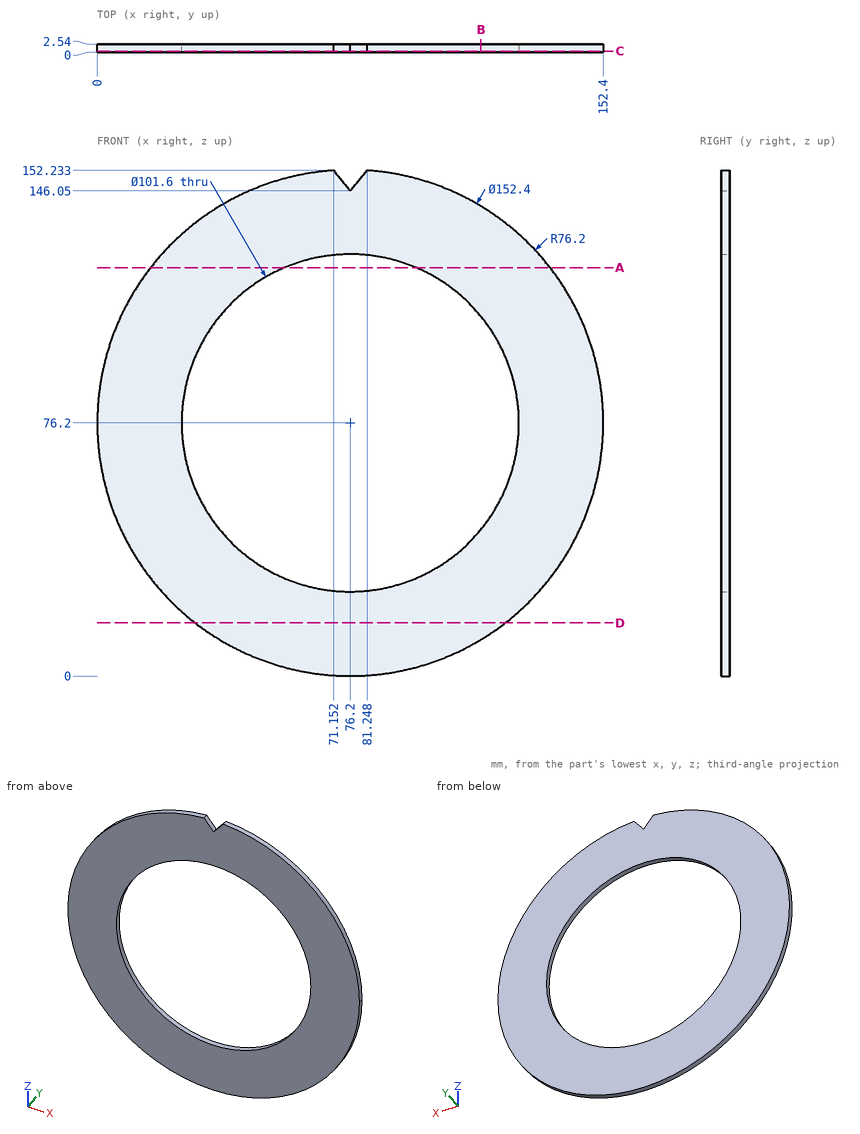
Print and shaded views of the part. All mm, measured from the part's lowest x, y and z. Round coordinates to 2 decimals unless told otherwise and drop trailing zeros. Write each loop counter-clockwise with the first axis right and the second up, starting at its lowest first coordinate (ties: lowest second). Pieces come first, ordered by that corner, then holes. Notation, with made-up numbers: (29.5, 82) - (84.5, 82) arc R32 cw to (84.5, 112) - close; hole circle Ø11 at (29, -17.5). An arc over 180 degrees is marked (long way). Use CSV: the item, a comma, the result in double quotes. Start each with the question number.
Item 1: Band-saw the part on A-A (z = 123). Write the cut outline in (x, y) (1 decimal).
Item 2: Band-saw the part on C-C (y = 0.4). Write the cut outline in (x, z), and give its area (3 significant figures).
Item 3: Band-saw the part on B-B (x = 115.5). Write the cut outline in (y, z).
Item 4: Drill centre lines: L1, parallel to Z at x = 76.2, y = 1.45; L2, parallel to X at y = 1.2, z = 118; L3, parallel to X at y = 1.55, z = 33.5 (1 decimal). Where is each one in solid material? Low to high. Write a range as [from, to].
Item 5: Band-saw the part on D-D (z = 16). Write the cut outline in (x, y), and give its area (3 significant figures).
Item 6: Pin check, flat tips, straight feed: P1, Ø1.5, axis at y = 0.5, z = 54.5, coming from the -X side; P2, Ø1.5, axis at x = 126.5, y = 1, coming from the +Z side; P3, Ø10, axis at x = 93.5, z = 115, coming from the +Y side. Stop position of each tip, or through.
Checked values:
1,outline,"(16.1, 0) - (56.4, 0) - (56.4, 2.5) - (16.1, 2.5) - close; (96, 0) - (136.3, 0) - (136.3, 2.5) - (96, 2.5) - close"
2,outline,"(71.15, 152.23) arc R76.2 ccw (long way) to (81.25, 152.23) - (76.2, 146.05) - close; hole circle Ø101.6 at (76.2, 76.2)"
2,area,"10,100 mm²"
3,outline,"(0, 10.92) - (2.54, 10.92) - (2.54, 44.01) - (0, 44.01) - close; (0, 108.39) - (2.54, 108.39) - (2.54, 141.48) - (0, 141.48) - close"
4,L1,"z = [0, 25.4], [127, 146.05]"
4,L2,"x = [12.49, 47.33], [105.07, 139.91]"
4,L3,"x = [13.1, 48.7], [103.7, 139.3]"
5,outline,"(29.48, 0) - (122.92, 0) - (122.92, 2.54) - (29.48, 2.54) - close"
5,area,"237 mm²"
6,P1,"stops at x = 2.94"
6,P2,"stops at z = 134.09"
6,P3,"passes through"
